Verification items for the finished model (mm, model axes). A direction names the side the tool comes from. Round coordinates to 2 decimals unless told otherwise and drop trailing zeros. Write each loop counter-clockwise with the first axis right and the second up, starting at its lowest first coordinate (ties: lowest second). Pieces come first, ordered by that corner, then holes. Notation, with made-up numbers: (64, 41.25) - (104, 41.25) arc R21 cw to (104, 68.25) - close; hole circle Ø1 at (6, 3.5). An arc over 180 degrees is marked (long way). Answer as a JSON object with one key per item and string values. Group by question number.
1) Section check B-B (z = 0). Enter the section's corners in (x, y).
2) Thickness scan on line 1 (X direction, y = 2.25, z = -7); line 2 (X direction, y = 1.1, z = 0); line 3 (Z direction, x = 1.25, y = 1.15). Record the ranges inside material, lowest first.
3) Set-up check for faces 1 (the flat face through (0, 2, 0)), 2 (the cylindrical face through (0, 1, 11)), 3 (the flat face through (0, 0, 7)): record each of +Z, -Z, +X, -X, +Y, -Y from which the full face is reachable in a straight line by a thin tool's end or side.
4) Mould release check, pull along X, two halves, no side actions. Record for faces 4 (the cylindrical face through (0.225, 0.732, -0.715)), 5 (the flat face through (-4, 1, 0)), 6 (the cylindrical face through (0, 1, -11)), 7 (the flat face through (4, 1, 0)): +X half, -X half, draft (parallel to the pull), parting line (faces both ways), or undercut.
5) Section check A-A (y = 0.75). Enter the section's corners in (x, z), then the cut area to 3 significant figures.
6) Go/stop test with flat-tipped pins: pin 1 Ø1.8 at (x, z) = (-1.5, -6.5) entering from +Y; pin 2 Ø1 at (x, y) = (3, 2.5) entering from +Z; pin 3 Ø1.2 at (x, z) = (-0.5, 0) entering from -Y; pin 4 Ø0.9 at (x, z) = (0, 0) entering from -Y. Record where each tip stops, or that it passes through.
7) Section check C-C (y = -0.3). Enter the section's corners in (x, z), then the cut area to 3 significant figures.
8) Section check D-D (x = 0). Enter the section's corners in (y, z).
```python
from build123d import *

# Parameters (mm, degrees)
SKETCH1_R           = 3
BOSS_EXTRUDE1_DEPTH = 3
BOSS_EXTRUDE2_START = 0.5
BOSS_EXTRUDE2_DEPTH = 0.5
SKETCH3_R           = 0.75
CUT_EXTRUDE1_DEPTH  = 2.5


with BuildPart() as part:
    # Sketch1 → Boss-Extrude1 (new body)
    with BuildSketch(Plane(origin=(0, 0, 0), x_dir=(1, 0, 0), z_dir=(0, 1, 0))):
        with BuildLine():
            Line((4, 7), (4, -7))
            ThreePointArc((4, -7), (0, -11), (-4, -7))
            Line((-4, -7), (-4, 7))
            ThreePointArc((-4, 7), (0, 11), (4, 7))
        make_face()
        with Locations(Location((0, 7, 0), (0, 0, 270))):
            Circle(SKETCH1_R, mode=Mode.SUBTRACT)
        with Locations(Location((0, -7, 0), (0, 0, 270))):
            Circle(SKETCH1_R, mode=Mode.SUBTRACT)
    extrude(amount=BOSS_EXTRUDE1_DEPTH)

    # Sketch2 → Boss-Extrude2 (add)
    with BuildSketch(Plane.XZ.offset(BOSS_EXTRUDE2_START)):
        with BuildLine():
            Line((4, 7), (4, -7))
            ThreePointArc((4, -7), (0, -11), (-4, -7))
            Line((-4, -7), (-4, 7))
            ThreePointArc((-4, 7), (0, 11), (4, 7))
        make_face()
    extrude(amount=-BOSS_EXTRUDE2_DEPTH)

    # Sketch3 → Cut-Extrude1 (cut)
    with BuildSketch(Plane.XZ.offset(0.5)):
        with Locations(Location((0, 0, 0), (0, 0, 270))):
            Circle(SKETCH3_R)
    extrude(amount=-CUT_EXTRUDE1_DEPTH, mode=Mode.SUBTRACT)


solid = part.part
```
Returned:
{
 "1": {"outline": "(-4, -0.5) - (-0.75, -0.5) - (-0.75, 2) - (0.75, 2) - (0.75, -0.5) - (4, -0.5) - (4, 3) - (-4, 3) - close"},
 "2": {"line 1": "-4 to -3, 3 to 4", "line 2": "-4 to -0.75, 0.75 to 4", "line 3": "-10.8 to -9.73, -4.27 to 4.27, 9.73 to 10.8"},
 "3": {"face 1": "-Y", "face 2": "+Z, +Y, -Y", "face 3": "+Y"},
 "4": {"face 4": "undercut", "face 5": "-X half", "face 6": "parting line", "face 7": "+X half"},
 "5": {"outline": "(-4, -7) arc R4 ccw to (4, -7) - (4, 7) arc R4 ccw to (-4, 7) - close; hole circle Ø6 at (0, -7); hole circle Ø6 at (0, 7); hole circle Ø1.5 at (0, 0)", "area": "104 mm2"},
 "6": {"pin 1": "y = 0", "pin 2": "z = 10.12", "pin 3": "y = -0.5", "pin 4": "y = 2"},
 "7": {"outline": "(-4, -7) arc R4 ccw to (4, -7) - (4, 7) arc R4 ccw to (-4, 7) - close; hole circle Ø1.5 at (0, 0)", "area": "160 mm2"},
 "8": {"outline": "(-0.5, -11) - (3, -11) - (3, -10) - (0, -10) - (0, -4) - (3, -4) - (3, 4) - (0, 4) - (0, 10) - (3, 10) - (3, 11) - (-0.5, 11) - (-0.5, 0.75) - (2, 0.75) - (2, -0.75) - (-0.5, -0.75) - close"}
}
